Can you work these out from the model? Positions are in its coordinate system, mm. A direction names the side the tool comes from. Give positions to 0.01 mm unless a question says otherwise; leave off trailing zeros. Order: outer loops, then holes, each group sorted by start corner. A loop starts at its lowest first (then second) coordinate and runs counter-clockwise, first axis right, second up. Notation, with made-up numbers: (9, -8) -> (49, -8) arc R6 cw to (49, -1) -> close; hole circle Ø7 at (55.5, -22). An arc over 180 degrees is marked (long way). Answer as a JSON object with one key per item and string values.
```python
from build123d import *

# Parameters (mm, degrees)
F0_R     = 9.525
F1_DEPTH = 50.8
F2_R     = 6.35
F3_SIZE  = 6.35


with BuildPart() as f1:
    # F0 (on Front) → F1 (new body)
    with BuildSketch(Plane.XZ):
        with BuildLine():
            Line((0, 25.4), (0, 0))
            Line((0, 0), (50.8, 0))
            ThreePointArc((50.8, 0), (68.760512, 43.360512), (25.4, 25.4))
            Line((25.4, 25.4), (0, 25.4))
        make_face()
        with Locations((50.8, 25.4)):
            Circle(F0_R, mode=Mode.SUBTRACT)
    extrude(amount=-F1_DEPTH)

    # F2
    f2_edges = [f1.edges().sort_by_distance(p)[0] for p in [
        (25.4, 25.4, 25.4),
    ]]
    fillet(f2_edges, radius=F2_R)

    # F3
    f3_edges = [f1.edges().sort_by_distance(p)[0] for p in [
        (0, 25.4, 0),
    ]]
    chamfer(f3_edges, length=F3_SIZE)


solid = f1.part
```
1. If we section it at B-B on x = 56.5: Please give me the cut outline in (y, z), then the cut area to 3 significant figures.
Worked answers:
{"outline": "(0, 0.65) -> (50.8, 0.65) -> (50.8, 17.77) -> (0, 17.77) -> close; (0, 33.03) -> (50.8, 33.03) -> (50.8, 50.15) -> (0, 50.15) -> close", "area": "1,740 mm²"}
2. Will these pins go through, and if not, where does the flat tip stop? pin 1 Ø1 at (x, y) = (14.5, 13) entering from +Z; pin 2 Ø1 at (y, z) = (40, 38.5) entering from -X; pin 3 Ø1.5 at (y, z) = (20.5, 33.5) entering from -X; pin 4 Ø17 at (x, z) = (50.8, 25.4) entering from +Y.
Worked answers:
{"pin 1": "z = 25.4", "pin 2": "x = 28.75", "pin 3": "x = 26.49", "pin 4": "through"}
3. Please list where these lines run through material, in increasing order: L1, parallel to Z at x = 50.8, y = 14.5 (3 decimals); L2, parallel to X at y = 36, z = 25; L3, parallel to X at y = 8, z = 24.
Worked answers:
{"L1": "0 to 15.875, 34.925 to 50.8", "L2": "0 to 41.28, 60.32 to 76.2", "L3": "0 to 41.38, 60.22 to 76.16"}
4. For faces 1 (the face through (10, 25, 25.4)), 2 (the face through (38, 0, 20)), which set-ups out of +Z, -Z, +X, -X, +Y, -Y let a thin tool reach every point of the face, with its end or its side?
Worked answers:
{"face 1": "+Z, -X, +Y, -Y", "face 2": "+Z, -Z, +X, -X, -Y"}
5. If we section it at C-C on z = 29.5: Please give me the cut outline in (x, y), then the cut area to 3 significant figures.
Worked answers:
{"outline": "(25.63, 0) -> (42.2, 0) -> (42.2, 50.8) -> (25.63, 50.8) -> close; (59.4, 0) -> (75.87, 0) -> (75.87, 50.8) -> (59.4, 50.8) -> close", "area": "1,680 mm²"}
6. If we section it at A-A on y = 16: Please give me the cut outline in (x, z) (3 decimals).
Worked answers:
{"outline": "(0, 6.35) -> (6.35, 0) -> (50.8, 0) arc R25.4 ccw (long way) to (25.913, 30.48) arc R6.35 cw to (19.691, 25.4) -> (0, 25.4) -> close; hole circle Ø19.05 at (50.8, 25.4)"}
7. If we mould it in two halves opening along Z, with no side actions, what happens to faces 3 (the face through (55.2, 25.04, 16.95)), 4 (the face through (23.66, 25.756, 26.793)), 5 (the face through (38, 50.8, 20)), 6 (the face through (28, 25, 0))? For each: +Z half, -Z half, draft (parallel to the pull), parting line (faces both ways), or undercut.
Worked answers:
{"face 3": "undercut", "face 4": "+Z half", "face 5": "draft", "face 6": "-Z half"}
8. If we section it at D-D on x = 15: Please give me the cut outline in (y, z).
Worked answers:
{"outline": "(0, 0) -> (50.8, 0) -> (50.8, 25.4) -> (0, 25.4) -> close"}
